```python
from build123d import *

# Parameters (mm, degrees)
SKETCH1_W                 = 98
SKETCH1_H                 = 99
MAIN_BODY_DEPTH           = 2
SKETCH2_R                 = 1.75
FRONTBACKBOLTHOLES_DEPTH  = 140.316187143
SKETCH3_R                 = 1.75
SIDEBOLTHOLES_DEPTH       = 140.316187143
M3X0_5_TAPPED_HOLE1_D     = 2.5
M3X0_5_TAPPED_HOLE1_DEPTH = 7.5
M3X0_5_TAPPED_HOLE1_TIP   = 0.751075774
SKETCH7_W                 = 9
SKETCH7_H                 = 13.5
CUT_EXTRUDE3_DEPTH        = 140.316187143
FILLET1_R                 = 4
SKETCH8_W                 = 60
SKETCH8_H                 = 3
BOSS_EXTRUDE2_DEPTH       = 2
SKETCH9_W                 = 3
SKETCH9_H                 = 60
BOSS_EXTRUDE3_DEPTH       = 2
CUT_EXTRUDE5_DEPTH        = 140.316187143


with BuildPart() as part:
    # Sketch1 → Main Body (new body)
    with BuildSketch(Plane.XY):
        with Locations((49, 49.5)):
            Rectangle(SKETCH1_W, SKETCH1_H)
    extrude(amount=MAIN_BODY_DEPTH)

    # Sketch2 → FrontBackBoltHoles (cut, through all)
    with BuildSketch(Plane.XY.offset(2)):
        with Locations((4, 82)):
            Circle(SKETCH2_R)
        with Locations((94, 82)):
            Circle(SKETCH2_R)
        with Locations((94, 17)):
            Circle(SKETCH2_R)
        with Locations((4, 17)):
            Circle(SKETCH2_R)
    extrude(amount=-FRONTBACKBOLTHOLES_DEPTH, mode=Mode.SUBTRACT)

    # Sketch3 → SideBoltHoles (cut, through all)
    with BuildSketch(Plane.XY.offset(2)):
        with Locations((21, 96)):
            Circle(SKETCH3_R)
        with Locations((77, 96)):
            Circle(SKETCH3_R)
        with Locations((77, 3)):
            Circle(SKETCH3_R)
        with Locations((21, 3)):
            Circle(SKETCH3_R)
    extrude(amount=-SIDEBOLTHOLES_DEPTH, mode=Mode.SUBTRACT)

    # M3x0.5 Tapped Hole1
    with Locations(Plane.XY.offset(2)):
        with Locations((12.5, 91.5), (85.5, 91.5), (85.5, 7.5), (12.5, 7.5), (35, 49.5), (63, 49.5)):
            Hole(M3X0_5_TAPPED_HOLE1_D / 2, depth=M3X0_5_TAPPED_HOLE1_DEPTH)
            with Locations((0, 0, -(M3X0_5_TAPPED_HOLE1_DEPTH + M3X0_5_TAPPED_HOLE1_TIP / 2))):  # 118° drill point
                Cone(0, M3X0_5_TAPPED_HOLE1_D / 2, M3X0_5_TAPPED_HOLE1_TIP, mode=Mode.SUBTRACT)

    # Sketch7 → Cut-Extrude3 (cut, through all)
    with BuildSketch(Plane.XY.offset(2)):
        with Locations((4.5, 92.25)):
            Rectangle(SKETCH7_W, SKETCH7_H)
        with Locations((93.5, 92.25)):
            Rectangle(SKETCH7_W, SKETCH7_H)
        with Locations((93.5, 6.75)):
            Rectangle(SKETCH7_W, SKETCH7_H)
        with Locations((4.5, 6.75)):
            Rectangle(SKETCH7_W, SKETCH7_H)
    extrude(amount=-CUT_EXTRUDE3_DEPTH, mode=Mode.SUBTRACT)

    # Fillet1
    fillet1_edges = [part.edges().sort_by_distance(p)[0] for p in [
        (89, 85.5, 1),
        (9, 13.5, 1),
        (89, 13.5, 1),
        (9, 85.5, 1),
    ]]
    fillet(fillet1_edges, radius=FILLET1_R)

    # Sketch8 → Boss-Extrude2 (add)
    with BuildSketch(Plane(origin=(0, 0, 0), x_dir=(-1, 0, 0), z_dir=(0, 0, -1))):
        with Locations((-49, 92)):
            Rectangle(SKETCH8_W, SKETCH8_H)
        with Locations((-49, 7)):
            Rectangle(SKETCH8_W, SKETCH8_H)
    extrude(amount=BOSS_EXTRUDE2_DEPTH)

    # Sketch9 → Boss-Extrude3 (add)
    with BuildSketch(Plane(origin=(0, 0, 0), x_dir=(-1, 0, 0), z_dir=(0, 0, -1))):
        with Locations((-89, 49.5)):
            Rectangle(SKETCH9_W, SKETCH9_H)
        with Locations((-9, 49.5)):
            Rectangle(SKETCH9_W, SKETCH9_H)
    extrude(amount=BOSS_EXTRUDE3_DEPTH)

    # Sketch11 → Cut-Extrude5 (cut, through all)
    with BuildSketch(Plane(origin=(0, 0, 0), x_dir=(-1, 0, 0), z_dir=(0, 0, -1))):
        with BuildLine():
            Line((-10.5, 37), (-10.5, 62))
            ThreePointArc((-10.5, 62), (-11.085786438, 63.414213562), (-12.5, 64))
            ThreePointArc((-12.5, 64), (-13.914213562, 63.414213562), (-14.5, 62))
            Line((-14.5, 62), (-14.5, 37))
            ThreePointArc((-14.5, 37), (-13.914213562, 35.585786438), (-12.5, 35))
            ThreePointArc((-12.5, 35), (-11.085786438, 35.585786438), (-10.5, 37))
        make_face()
        with BuildLine():
            ThreePointArc((-14.5, 62), (-13.914213562, 63.414213562), (-12.5, 64))
            Line((-12.5, 64), (-21, 64))
            ThreePointArc((-21, 64), (-19.585786438, 63.414213562), (-19, 62))
            Line((-19, 62), (-19, 37))
            ThreePointArc((-19, 37), (-19.585786438, 35.585786438), (-21, 35))
            Line((-21, 35), (-12.5, 35))
            ThreePointArc((-12.5, 35), (-13.914213562, 35.585786438), (-14.5, 37))
            Line((-14.5, 37), (-14.5, 62))
        make_face()
        with BuildLine():
            Line((-23, 62), (-23, 37))
            ThreePointArc((-23, 37), (-21, 35), (-19, 37))
            Line((-19, 37), (-19, 62))
            ThreePointArc((-19, 62), (-21, 64), (-23, 62))
        make_face()
    extrude(amount=-CUT_EXTRUDE5_DEPTH, mode=Mode.SUBTRACT)


solid = part.part
```
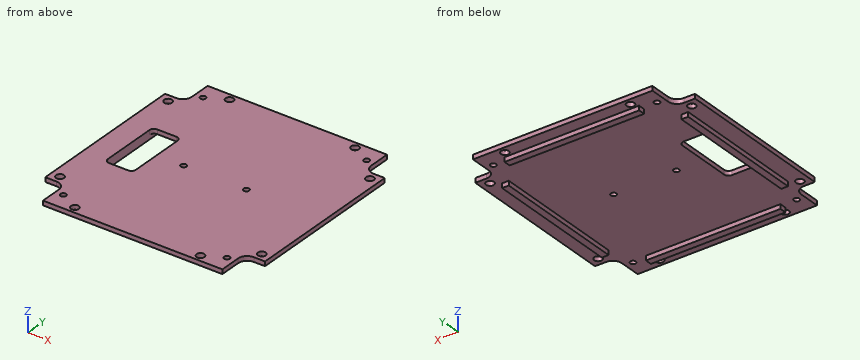
Could you check a few things on this model? Use its own coordinates, in mm. Give positions to 0.01 mm unless a question says otherwise; leave off trailing zeros. Order: outer loops, then holes, each group sorted by start corner. A loop starts at its lowest first (then second) coordinate and runs counter-clockwise, first axis right, second up.
Q1. Suppose I cut it at C-C, the plane y = 17. Write out the boundary of the cut face in (x, z).
Q2. Suppose I cut it at B-B, the plane x = 77. Write out the boundary of the cut face in (y, z), and give its area (3 significant figures).
Q3. If I drill on line 1 along Y through (x, z) = (21, 1.1); line 2 along X through (y, z) = (96, 0.45); line 3 along Y through (x, z) = (85.5, 1.1), over which ranges is the centre line in solid material (lowest first)?
Q4. I'm going to push flat-ended pins straight in: P1, Ø1.5, axis at x = 35, y = 49.5, coming from the -Z side; P2, Ø2, axis at x = 44.5, z = -1.5, coming from the -Y side; P3, Ø1, axis at x = 17, z = 0.5, coming from the -Y side; P4, Ø1.6, axis at y = 94, z = 1, coming from the +X side. Where does each tip first touch, or does it pass through?
Q5. Suppose I cut it at A-A, the plane y = 56. Write out the boundary of the cut face in (x, z), and give its area (3 significant figures).
Q6. Suppose I cut it at D-D, the plane x = 63. Write out the boundary of the cut face in (y, z), and give its area (3 significant figures).
Solution:
1. outline: (0, 0) - (2.25, 0) - (2.25, 2) - (0, 2) - close; (5.75, 0) - (92.25, 0) - (92.25, 2) - (5.75, 2) - close; (95.75, 0) - (98, 0) - (98, 2) - (95.75, 2) - close
2. outline: (0, 0) - (1.25, 0) - (1.25, 2) - (0, 2) - close; (4.75, 0) - (5.5, 0) - (5.5, -2) - (8.5, -2) - (8.5, 0) - (90.5, 0) - (90.5, -2) - (93.5, -2) - (93.5, 0) - (94.25, 0) - (94.25, 2) - (4.75, 2) - close; (97.75, 0) - (99, 0) - (99, 2) - (97.75, 2) - close
2. area: 196 mm2
3. line 1: y = 0 to 1.25, 4.75 to 35, 64 to 94.25, 97.75 to 99
3. line 2: x = 9 to 19.25, 22.75 to 75.25, 78.75 to 89
3. line 3: y = 0 to 6.25, 8.75 to 90.25, 92.75 to 99
4. P1: passes through
4. P2: stops at y = 5.5
4. P3: stops at y = 0
4. P4: stops at x = 89
5. outline: (0, 0) - (7.5, 0) - (7.5, -2) - (10.5, -2) - (10.5, 2) - (0, 2) - close; (23, 0) - (87.5, 0) - (87.5, -2) - (90.5, -2) - (90.5, 0) - (98, 0) - (98, 2) - (23, 2) - close
5. area: 183 mm2
6. outline: (0, 0) - (5.5, 0) - (5.5, -2) - (8.5, -2) - (8.5, 0) - (48.25, 0) - (48.25, 2) - (0, 2) - close; (50.75, 0) - (90.5, 0) - (90.5, -2) - (93.5, -2) - (93.5, 0) - (99, 0) - (99, 2) - (50.75, 2) - close
6. area: 205 mm2
